Can you work these out from the drawing? Everything is in mm from the part's minimum corner. Coordinates: 2 decimals unless noted, no trailing zeros. Order: outer loops, then holes, each group sorted by start corner. A loop starts at its lowest first (then second) coordinate and runs counter-clockwise, first axis right, second up. Notation, with made-up numbers: (16, -28) -> (62, -28) arc R10 ccw to (62, -10) -> close; hole circle Ø3 at (-3, 65.5). An arc over 180 degrees is marked (long way). Return JSON: item names as keys, results as strings. Group by question number.
1) For pin 1 (2 mm diameter, centred on x = 14, z = 7, fed in from -Y), with a flat end and sliding along its axis, tell me the tip position at first contact or that it passes through.
2) If we section it at B-B, the plane z = 5.5: Please give me the cut outline in (x, y) (3 decimals).
3) Thinking about a two-plate mould opening in X: for the marked faces 1, 2 and 3, which applies, +X half, -X half, draft (parallel to the pull), parting line (faces both ways), or undercut?
4) If I drill on probe 1 along Y at (x, z) = (9.5, 16.25); probe 2 along Z at (x, y) = (15, 8); probe 3 along Y at (x, z) = (8.25, 6.5), over which ranges is the centre line in solid material (lowest first)? Write a range as from..to.
5) If we section it at A-A, the plane z = 13: Please give me the cut outline in (x, y) (3 decimals), then the cut area to 3 significant figures.
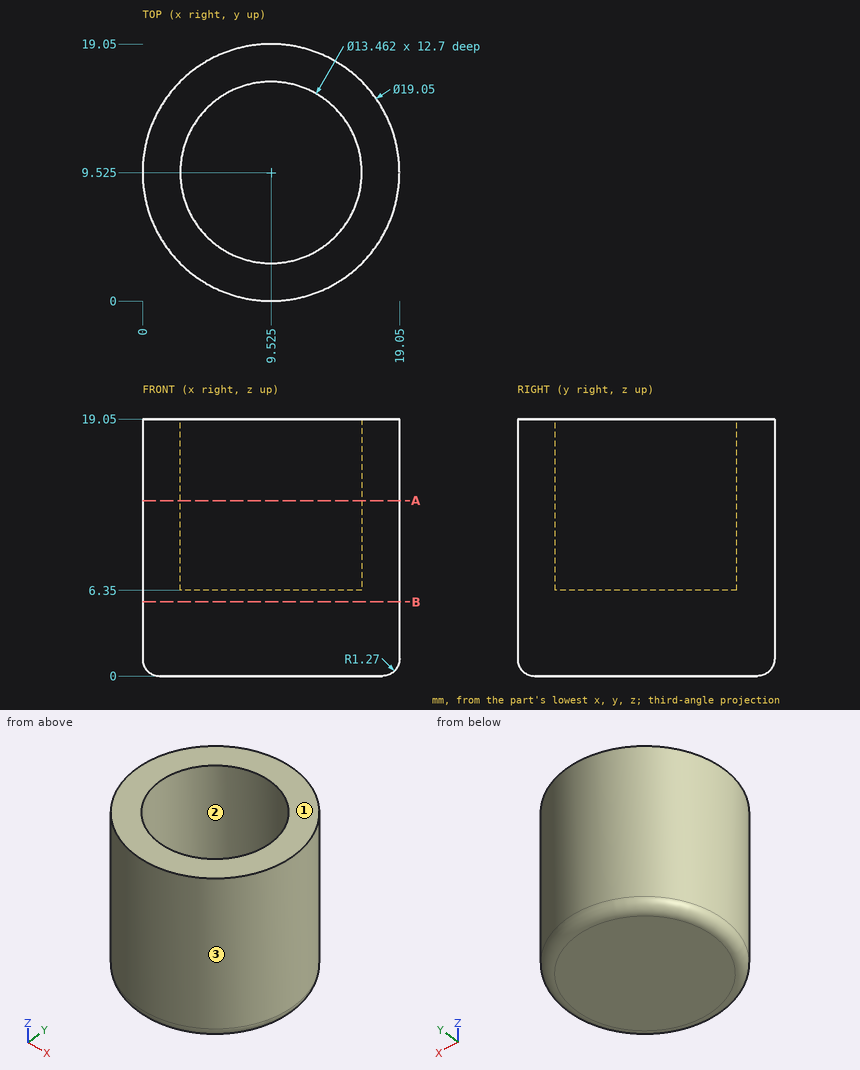
Result sheet:
{
 "1": {"pin 1": "stops at y = 0.66"},
 "2": {"outline": "circle Ø19.05 at (9.525, 9.525)"},
 "3": {"face 1": "draft", "face 2": "undercut", "face 3": "parting line"},
 "4": {"probe 1": "y = 0..2.79, 16.26..19.05", "probe 2": "z = 0..6.35", "probe 3": "y = 0.09..2.92, 16.13..18.96"},
 "5": {"outline": "circle Ø19.05 at (9.525, 9.525); hole circle Ø13.462 at (9.525, 9.525)", "area": "143 mm2"}
}
